```python
from build123d import *

# Parameters (mm, degrees)
SKETCH_1_R          = 10
EXTRUDE_1_DEPTH     = 2
SKETCH_2_R          = 3.5
EXTRUDE_2_DEPTH     = 1
SKETCH_3_R          = 6
EXTRUDE_3_DEPTH     = 9
SKETCH_4_R          = 4
EXTRUDE_4_DEPTH     = 3
SKETCH_5_R          = 3
EXTRUDE_5_DEPTH     = 6
EXTRUDE_START       = 35
SKETCH_6_R          = 3
EXTRUDE_6_DEPTH     = 35
EXTRUDE_START_2     = 1
SKETCH_7_R          = 3.5
EXTRUDE_7_DEPTH     = 1
EXTRUDE_START_3     = 9
SKETCH_8_R          = 3
EXTRUDE_8_DEPTH     = 9
SKETCH_9_R          = 2
EXTRUDE_9_DEPTH     = 5
CHAMFER_1_SIZE      = 0.5
SKETCH_11_W         = 4
SKETCH_11_H         = 0.3
CUT_EXTRUDE_2_DEPTH = 5
CUT_EXTRUDE_START   = 2
SKETCH_12_R         = 6
SKETCH_12_R_2       = 4.5
CUT_EXTRUDE_3_DEPTH = 1
CUT_EXTRUDE_START_2 = -6
SKETCH_13_R         = 6
SKETCH_13_R_2       = 5
CUT_EXTRUDE_4_DEPTH = 6
SKETCH_15_R         = 3
SKETCH_15_R_2       = 2.9
CUT_EXTRUDE_5_DEPTH = 3


with BuildPart() as part:
    # 草图1 → 凸台-拉伸1 (new body)
    with BuildSketch(Plane(origin=(0, 0, 0), x_dir=(0, 0, -1), z_dir=(1, 0, 0))):
        Circle(SKETCH_1_R)
    extrude(amount=EXTRUDE_1_DEPTH)

    # 草图2 → 凸台-拉伸2 (add)
    with BuildSketch(Plane(origin=(2, 0, 0), x_dir=(0, 0, -1), z_dir=(1, 0, 0))):
        Circle(SKETCH_2_R)
    extrude(amount=EXTRUDE_2_DEPTH)

    # 草图3 → 凸台-拉伸3 (add)
    with BuildSketch(Plane.ZY):
        with Locations(Location((0, 0, 0), (0, 0, 180))):
            Circle(SKETCH_3_R)
    extrude(amount=EXTRUDE_3_DEPTH)

    # 草图4 → 凸台-拉伸4 (add)
    with BuildSketch(Plane.ZY.offset(9)):
        Circle(SKETCH_4_R)
    extrude(amount=EXTRUDE_4_DEPTH)

    # 草图5 → 凸台-拉伸5 (add)
    with BuildSketch(Plane(origin=(3, 0, 0), x_dir=(0, 0, -1), z_dir=(1, 0, 0))):
        Circle(SKETCH_5_R)
    extrude(amount=EXTRUDE_5_DEPTH)

    # 草图6 → 凸台-拉伸6 (add)
    with BuildSketch(Plane.ZY.offset(12).offset(EXTRUDE_START)):
        with Locations(Location((0, 0, 0), (0, 0, 180))):
            Circle(SKETCH_6_R)
    extrude(amount=-EXTRUDE_6_DEPTH)

    # 草图7 → 凸台-拉伸7 (add)
    with BuildSketch(Plane.ZY.offset(47).offset(EXTRUDE_START_2)):
        with Locations(Location((0, 0, 0), (0, 0, 180))):
            Circle(SKETCH_7_R)
    extrude(amount=-EXTRUDE_7_DEPTH)

    # 草图8 → 凸台-拉伸8 (add)
    with BuildSketch(Plane.ZY.offset(48).offset(EXTRUDE_START_3)):
        with Locations(Location((0, 0, 0), (0, 0, 180))):
            Circle(SKETCH_8_R)
    extrude(amount=-EXTRUDE_8_DEPTH)

    # 草图9 → 凸台-拉伸9 (add)
    with BuildSketch(Plane.ZY.offset(57)):
        Circle(SKETCH_9_R)
    extrude(amount=EXTRUDE_9_DEPTH)

    # 倒角1
    chamfer_1_edges = [part.edges().sort_by_distance(p)[0] for p in [
        (9, 0, 3),
    ]]
    chamfer(chamfer_1_edges, length=CHAMFER_1_SIZE)

    # 草图11 → 切除-拉伸2 (cut, symmetric)
    with BuildSketch(Plane(origin=(0, 0, 0), x_dir=(1, 0, 0), z_dir=(0, 1, 0))):
        with Locations((-44, 2.85)):
            Rectangle(SKETCH_11_W, SKETCH_11_H)
        with Locations((-44, -2.85)):
            Rectangle(SKETCH_11_W, SKETCH_11_H)
    extrude(amount=CUT_EXTRUDE_2_DEPTH, both=True, mode=Mode.SUBTRACT)

    # 草图12 → 切除-拉伸3 (cut)
    with BuildSketch(Plane.ZY.offset(CUT_EXTRUDE_START)):
        Circle(SKETCH_12_R)
        Circle(SKETCH_12_R_2, mode=Mode.SUBTRACT)
    extrude(amount=CUT_EXTRUDE_3_DEPTH, mode=Mode.SUBTRACT)

    # 草图13 → 切除-拉伸4 (cut)
    with BuildSketch(Plane.ZY.offset(9).offset(CUT_EXTRUDE_START_2)):
        with Locations(Location((0, 0, 0), (0, 0, 180))):
            Circle(SKETCH_13_R)
        Circle(SKETCH_13_R_2, mode=Mode.SUBTRACT)
    extrude(amount=CUT_EXTRUDE_4_DEPTH, mode=Mode.SUBTRACT)

    # 草图14 → 旋转1 (revolve)
    with BuildSketch(Plane.XY, mode=Mode.PRIVATE) as revolve_1_sk:
        Polygon((-12, 4), (-17, 3), (-12, 3), align=None)
    revolve(revolve_1_sk.sketch.rotate(Axis((-6.238584256, 0, 0), (-1, 0, 0)), 90), axis=Axis((-6.238584256, 0, 0), (-1, 0, 0)))

    # 草图15 → 切除-拉伸5 (cut)
    with BuildSketch(Plane.ZY.offset(57)):
        Circle(SKETCH_15_R)
        Circle(SKETCH_15_R_2, mode=Mode.SUBTRACT)
    extrude(amount=-CUT_EXTRUDE_5_DEPTH, mode=Mode.SUBTRACT)


solid = part.part
```
Geometry: final body of the model. Coordinates: model frame, mm. A direction names the side the tool comes from. Give positions to 0.01 mm unless a question says otherwise; leave off trailing zeros. Write each loop counter-clockwise with the first axis right and the second up, starting at its lowest first coordinate (ties: lowest second). Pieces come first, ordered by that corner, then holes.
1. Section query B-B, the plane x = -34. Return loops of the section in (y, z), then the cut area to 3 significant figures.
2. Reachability of faces 1 (the flat face through (-44, 0, -2.7)), 2 (the cylindrical face through (-10.479, -3.905, -0.867)), 3 (the cylindrical face through (2.493, -1.341, -3.233)) from +Z, -Z, +X, -X, +Y, -Y: full face, straight path, thin tool, end or side. Return the list, or none.
3. Section query A-A, the plane y = -8. Return loops of the section in (x, z).
4. Section query C-C, the plane y = 8.5. Return loops of the section in (x, z), then the cut area to 3 significant figures.
5. Line query: probe 1 along X at (y, z) = (-4.5, 2); probe 2 along X at (y, z) = (-7.5, 3.25); probe 3 along Y at (x, z) = (-44, -0.75). Output: solid intervals per line, ascending.
6. Draft query along X for faces 4 (the flat face through (0, -7, 0)), 5 (the flat face through (-2, 4.5, -1.4)), 6 (the flat face through (9, 0, 0)), 7 (the cylindrical face through (-5.96, -4.88, -1.08)). Return one class per face: released by +X, released by -X, zero draft, split by the parting line, or undercut.
7. Pin query (flat end, axial travel): P1, Ø6, axis at x = -41, z = 4.5, coming from the +Y side; P2, Ø3.5, axis at y = 0.5, z = -2, coming from the -X side; P3, Ø2, axis at x = -12.5, z = 4, coming from the -Y side; P4, Ø1.5, axis at y = 7.5, z = 7, coming from the +X side. Return the tip coordinate at first contact, or that it passes through.
Computed:
1. outline: circle Ø6 at (0, 0)
1. area: 28.3 mm2
2. face 1: -Z, +Y, -Y
2. face 2: -X
2. face 3: +X
3. outline: (0, -6) - (2, -6) - (2, 6) - (0, 6) - close
4. outline: (0, -5.27) - (2, -5.27) - (2, 5.27) - (0, 5.27) - close
4. area: 21.1 mm2
5. probe 1: x = -9 to -3, -2 to 2
5. probe 2: x = 0 to 2
5. probe 3: y = -2.9 to 2.9
6. face 4: released by -X
6. face 5: undercut
6. face 6: released by +X
6. face 7: zero draft
7. P1: stops at y = 2.6
7. P2: stops at x = -62
7. P3: stops at y = -2.53
7. P4: stops at x = 2
